For this review, take the finished solid that the model builds, in its own axes (mm). Give positions to 0.01 mm unless a question says otherwise; leave off trailing zeros. Loops run counter-clockwise (first coordinate to the right, second up) from the corner with the lowest first, then second, coordinate; pieces in that order, holes last.
```python
from build123d import *

# Parameters (mm, degrees)
BOSS_EXTRUDE1_DEPTH = 23
CUT_EXTRUDE1_REACH  = 33.209
SKETCH2_R           = 2.6
CHAMFER1_SIZE       = 1


with BuildPart() as part:
    # Sketch1 → Boss-Extrude1 (new body)
    with BuildSketch(Plane(origin=(0, 0, 0), x_dir=(1, 0, 0), z_dir=(0, 1, 0))):
        with BuildLine():
            Line((-18, 0), (18, 0))
            Line((18, 0), (18, -11))
            Line((18, -11), (4.92449236, -11))
            ThreePointArc((4.92449236, -11), (0, -6.975), (-4.92449236, -11))
            Line((-4.92449236, -11), (-18, -11))
            Line((-18, -11), (-18, 0))
        make_face()
    extrude(amount=BOSS_EXTRUDE1_DEPTH)

    # Sketch2 → Cut-Extrude1 (cut, up to next)
    with BuildSketch(Plane.XY.offset(11), mode=Mode.PRIVATE) as cut_extrude1_sk1:
        with Locations((-12, 11.5)):
            Circle(SKETCH2_R)
    cut_extrude1_tool1 = extrude(cut_extrude1_sk1.sketch, amount=-CUT_EXTRUDE1_REACH, mode=Mode.PRIVATE) & part.part
    # Sketch2 → Cut-Extrude1 (cut, up to next)
    with BuildSketch(Plane.XY.offset(11), mode=Mode.PRIVATE) as cut_extrude1_sk2:
        with Locations((12, 11.5)):
            Circle(SKETCH2_R)
    cut_extrude1_tool2 = extrude(cut_extrude1_sk2.sketch, amount=-CUT_EXTRUDE1_REACH, mode=Mode.PRIVATE) & part.part
    add(cut_extrude1_tool1.solids().sort_by_distance((-12, 11.5, 11))[0], mode=Mode.SUBTRACT)
    add(cut_extrude1_tool2.solids().sort_by_distance((12, 11.5, 11))[0], mode=Mode.SUBTRACT)

    # Chamfer1
    chamfer1_edges = [part.edges().sort_by_distance(p)[0] for p in [
        (-18, 11.5, 0),
        (18, 11.5, 0),
        (18, 23, 5.5),
        (0, 23, 0),
        (-18, 23, 5.5),
        (0, 0, 0),
        (18, 0, 5.5),
        (-18, 0, 5.5),
    ]]
    chamfer(chamfer1_edges, length=CHAMFER1_SIZE)


solid = part.part
```
Item 1: For L1, parallel to Y at x = 12, z = 8.75; L2, parallel to X at y = 13, z = 0.5; L3, parallel to X at y = 7.75, z = 10.25, list the stretches that pass through material, from the lowest coordinate up.
Answer:
L1: y = 0 to 8.9, 14.1 to 23
L2: x = -17.5 to -14.12, -9.88 to 9.88, 14.12 to 17.5
L3: x = -18 to -4.71, 4.71 to 18
Item 2: Take a section at A-A on x = 12. Give the boundary of the cut face in (y, z).
Answer:
outline: (0, 1) - (1, 0) - (8.9, 0) - (8.9, 11) - (0, 11) - close; (14.1, 0) - (22, 0) - (23, 1) - (23, 11) - (14.1, 11) - close
Item 3: Take a section at C-C on z = 8.5. Give the boundary of the cut face in (x, y).
Answer:
outline: (-18, 1) - (-17, 0) - (-3.61, 0) - (-3.61, 23) - (-17, 23) - (-18, 22) - close; (3.61, 0) - (17, 0) - (18, 1) - (18, 22) - (17, 23) - (3.61, 23) - close; hole circle Ø5.2 at (-12, 11.5); hole circle Ø5.2 at (12, 11.5)
Item 4: Take a section at D-D on z = 3. Give the boundary of the cut face in (x, y).
Answer:
outline: (-18, 1) - (-17, 0) - (17, 0) - (18, 1) - (18, 22) - (17, 23) - (-17, 23) - (-18, 22) - close; hole circle Ø5.2 at (-12, 11.5); hole circle Ø5.2 at (12, 11.5)
Item 5: Clearance check with a flat-ended pin moving along its axis: pin 1 Ø5 at (x, y) = (-2, 3) entering from +Z. State where the tip first meets the part, or that it passes through.
Answer:
pin 1: stops at z = 9.76
Item 6: The part is to be moulded in two halves that separate along Y. For faces 1 (the flat face through (0, 0, 6)), 2 (the flat face through (-17.5, 11.4, 0.5)), 3 (the flat face through (17.3, 22.4, 0.7)), 4 (the cylindrical face through (13.2, 9.193, 5.577)), say which applies: released by +Y, released by -Y, zero draft, split by the parting line, or undercut.
Answer:
face 1: released by -Y
face 2: zero draft
face 3: released by +Y
face 4: undercut
Item 7: Take a section at B-B on y = 11.5. State how many separate pieces and enclosed holes the cut face has, and give its area (3 significant figures).
Answer:
separate pieces: 3
enclosed holes: 0
area: 251 mm2
